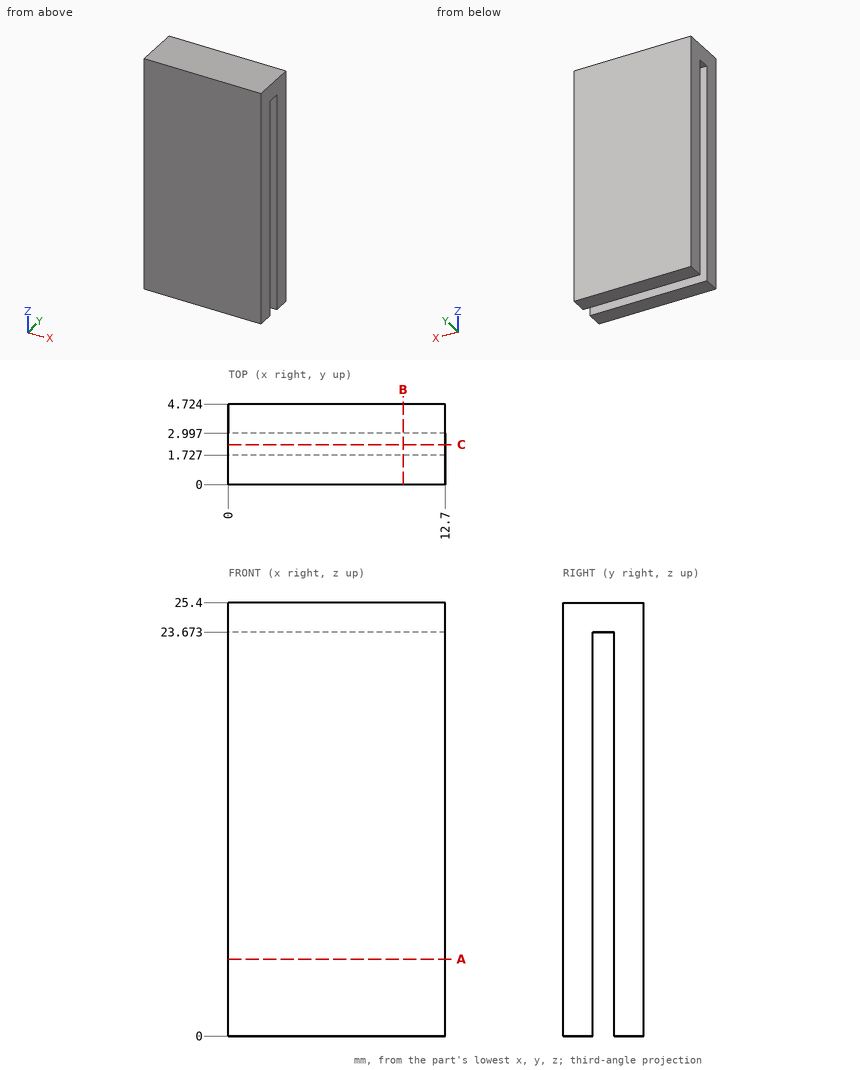
Study the drawing (mm; zero at the part's minimum x, y, z) and answer. Give positions to 0.01 mm unless a question says otherwise; leave off trailing zeros. Write each loop counter-clockwise with the first axis right and the second up, starting at its lowest first coordinate (ties: lowest second). Pieces come first, ordered by that corner, then holes.
Item 1: Find the intervals of material crossed by line 1 along Y through (x, z) = (2.25, 13.5) (1 decimal); line 2 along Z through (x, y) = (3, 2.95), in increasing order.
Item 2: Section B-B, the plane x = 10.25 is taken. Write down the section's boundary in (y, z) (1 decimal).
Item 3: Section C-C, the plane y = 2.35 is taken. Write down the section's boundary in (x, z).
Item 4: Section A-A, the plane z = 4.5 is taken. Write down the section's boundary in (x, y) (1 decimal).
Completed:
1. line 1: y = 0 to 1.7, 3 to 4.7
1. line 2: z = 23.67 to 25.4
2. outline: (0, 0) - (1.7, 0) - (1.7, 23.7) - (3, 23.7) - (3, 0) - (4.7, 0) - (4.7, 25.4) - (0, 25.4) - close
3. outline: (0, 23.67) - (12.7, 23.67) - (12.7, 25.4) - (0, 25.4) - close
4. outline: (0, 0) - (12.7, 0) - (12.7, 1.7) - (0, 1.7) - close; (0, 3) - (12.7, 3) - (12.7, 4.7) - (0, 4.7) - close
